The model under review builds one solid part; all positions refer to its coordinate system, in mm. A direction names the side the tool comes from. Give positions to 0.01 mm unless a question says otherwise; leave off trailing zeros. Write each loop counter-clockwise with the first axis right and the second up, starting at its lowest first coordinate (ties: lowest second). Pieces come first, ordered by that corner, then holes.
from build123d import *

# Parameters (mm, degrees)
BOSS_EXTRUDE1_DEPTH = 188


with BuildPart() as part:
    # Sketch2 → Boss-Extrude1 (new body)
    with BuildSketch(Plane(origin=(0, 0, 0), x_dir=(1, 0, 0), z_dir=(0, 1, 0))):
        with BuildLine():
            Line((-0.945896367, 0), (-54, 0))
            ThreePointArc((-54, 0), (-54.707106781, 0.292893219), (-55, 1))
            Line((-55, 1), (-55, 5))
            Line((-55, 5), (-2.487604379, 5))
            Line((-2.487604379, 5), (-2.487604379, 7.3))
            Line((-2.487604379, 7.3), (-37.487604379, 7.3))
            Line((-37.487604379, 7.3), (-37.487604379, 11.3))
            ThreePointArc((-37.487604379, 11.3), (-37.19471116, 12.007106781), (-36.487604379, 12.3))
            Line((-36.487604379, 12.3), (-4.82407147, 12.3))
            ThreePointArc((-4.82407147, 12.3), (-3.921954071, 12.438849148), (-3.103342161, 12.842543867))
            Line((-3.103342161, 12.842543867), (24.489595683, 32.163326947))
            ThreePointArc((24.489595683, 32.163326947), (25.236820297, 32.328982656), (25.882324164, 31.917751339))
            Line((25.882324164, 31.917751339), (28.176629909, 28.641143162))
            Line((28.176629909, 28.641143162), (-0.493691641, 8.56596789))
            Line((-0.493691641, 8.56596789), (0.825534163, 6.681918188))
            Line((0.825534163, 6.681918188), (42.185480254, 35.642464221))
            Line((42.185480254, 35.642464221), (44.479786, 32.365856044))
            ThreePointArc((44.479786, 32.365856044), (44.645441708, 31.61863143), (44.234210392, 30.973127563))
            Line((44.234210392, 30.973127563), (0.774832942, 0.542543867))
            ThreePointArc((0.774832942, 0.542543867), (-0.043778968, 0.138849148), (-0.945896367, 0))
        make_face()
    extrude(amount=BOSS_EXTRUDE1_DEPTH)


solid = part.part
1) To check wall thickness, follow probe 1 along Z at (x, y) = (-11, 93); probe 2 along X at (y, z) = (156, -14.5); probe 3 along X at (y, z) = (154, -7). State the ranges of each line that lie inside material, in increasing order.
2) Consider section A-A, the plane x = -21.5. Give the boundary of the cut face in (y, z).
3) Insertion check: pin 1 (0.7 mm diameter, centred on y = 136, z = -6, fed in from -X); pin 2 (10 mm diameter, centred on y = 44, z = -7.5, fed in from -X); pin 3 (6 mm diameter, centred on x = -20, y = 91.5, fed in from -Z); pin 4 (2 mm diameter, centred on y = 97, z = -29.5, fed in from +X). Each pin has a flat end and moves straight along its axis. Give the tip position at first contact, or say it passes through.
4) Consider section C-C, the plane z = -22. Give the boundary of the cut face in (x, y), then the cut area to 3 significant figures.
5) The part is to be moulded in two halves that separate along X. For faces 1 (the flat face through (10.5, 92.68, -22.37)), 2 (the flat face through (22.81, 92.68, -15.97)), 3 (the flat face through (14.042, 92.684, -18.744)), say which applies: +X half, -X half, draft (parallel to the pull), parting line (faces both ways), or undercut.
6) Consider section B-B, the plane y = 173. Give the boundary of the cut face in (x, z), then the cut area to 3 significant figures.
7) Consider section D-D, the plane z = -3. Give the boundary of the cut face in (x, y), then the cut area to 3 significant figures.
8) Tool access review of faces 4 (the flat face through (21.22, 92.68, -20.96)), 5 (the flat face through (43.317, 92.684, -34.027)), 6 (the flat face through (27.013, 92.684, -30.302)), 7 (the flat face through (-29, 93, -5)), 8 (the flat face through (-21, 93, -12.3)): name each direction out of +Z, -Z, +X, -X, +Y, -Y from which nothing blocks a thin tool from reaching the whole face with its end or side.
Answer block:
1. probe 1: z = -12.3 to -7.3, -5 to 0
1. probe 2: x = -0.74 to 7.98, 11.99 to 20.71
1. probe 3: x = -2.49 to 0.6, 1.28 to 10
2. outline: (0, -12.3) - (188, -12.3) - (188, -7.3) - (0, -7.3) - close; (0, -5) - (188, -5) - (188, 0) - (0, 0) - close
3. pin 1: stops at x = -2.49
3. pin 2: stops at x = -55
3. pin 3: stops at z = -12.3
3. pin 4: stops at x = 43.56
4. outline: (9.97, 0) - (18.69, 0) - (18.69, 188) - (9.97, 188) - close; (22.7, 0) - (31.42, 0) - (31.42, 188) - (22.7, 188) - close
4. area: 3,280 mm2
5. face 1: -X half
5. face 2: +X half
5. face 3: undercut
6. outline: (-55, -5) - (-2.49, -5) - (-2.49, -7.3) - (-37.49, -7.3) - (-37.49, -11.3) arc R1 ccw to (-36.49, -12.3) - (-4.82, -12.3) arc R3 cw to (-3.1, -12.84) - (24.49, -32.16) arc R1 ccw to (25.88, -31.92) - (28.18, -28.64) - (-0.49, -8.57) - (0.83, -6.68) - (42.19, -35.64) - (44.48, -32.37) arc R1 ccw to (44.23, -30.97) - (0.77, -0.54) arc R3 ccw to (-0.95, 0) - (-54, 0) arc R1 ccw to (-55, -1) - close
6. area: 903 mm2
7. outline: (-55, 0) - (4.28, 0) - (4.28, 188) - (-55, 188) - close
7. area: 11,100 mm2
8. face 4: +Y, -Y
8. face 5: -Z, +X, +Y, -Y
8. face 6: -Z, +Y, -Y
8. face 7: -X, +Y, -Y
8. face 8: -Z, -X, +Y, -Y
